Design review of the part built by this model. Coordinates are the model's own, in mm. Round coordinates to 2 decimals unless told otherwise and drop trailing zeros. Order: outer loops, then holes, each group sorted by start corner. A loop starts at its lowest first (then second) coordinate and runs counter-clockwise, first axis right, second up. Notation, with made-up numbers: (36, -1.5) - (41, -1.5) arc R21 ccw to (41, 2.5) - close; hole circle Ø3 at (-30, 40). An arc over 180 degrees is marked (long way). Write item = value, one per line.
from build123d import *

# Parameters (mm, degrees)
SKETCH_1_W                       = 385
SKETCH_1_H                       = 240
EXTRUDE_1_DEPTH                  = 16
SKETCH_2_R                       = 13.5
CUT_EXTRUDE_1_DEPTH              = 454.961452108
PATTERN_LINEAR_1_COUNT           = 2
PATTERN_LINEAR_1_PITCH           = 80
PATTERN_LINEAR_2_COUNT           = 2
PATTERN_LINEAR_2_PITCH           = 80
PATTERN_LINEAR_3_COUNT           = 2
PATTERN_LINEAR_3_PITCH           = 80
PATTERN_LINEAR_3_COPY_1_SKETCH_R = 13.5
PATTERN_LINEAR_3_COPY_1_DEPTH    = 454.961452108
PATTERN_LINEAR_3_COPY_2_SKETCH_R = 13.5
PATTERN_LINEAR_3_COPY_2_DEPTH    = 454.961452108
PATTERN_LINEAR_4_COUNT           = 2
PATTERN_LINEAR_4_PITCH           = 225
PATTERN_LINEAR_4_COPY_1_SKETCH_R = 13.5
PATTERN_LINEAR_4_COPY_1_DEPTH    = 454.961452108
PATTERN_LINEAR_4_COPY_2_SKETCH_R = 13.5
PATTERN_LINEAR_4_COPY_2_DEPTH    = 454.961452108
PATTERN_LINEAR_4_COPY_3_SKETCH_R = 13.5
PATTERN_LINEAR_4_COPY_3_DEPTH    = 454.961452108
PATTERN_LINEAR_4_COPY_4_SKETCH_R = 13.5
PATTERN_LINEAR_4_COPY_4_DEPTH    = 454.961452108
PATTERN_LINEAR_4_COPY_5_SKETCH_R = 13.5
PATTERN_LINEAR_4_COPY_5_DEPTH    = 454.961452108


with BuildPart() as part:
    # 草图1 → 凸台-拉伸1 (new body)
    with BuildSketch(Plane(origin=(0, 0, 0), x_dir=(1, 0, 0), z_dir=(0, 1, 0))):
        with Locations((192.5, 120)):
            Rectangle(SKETCH_1_W, SKETCH_1_H)
    extrude(amount=EXTRUDE_1_DEPTH)

    # 草图2 → 切除-拉伸1 (cut, through all)
    with BuildSketch(Plane(origin=(0, 16, 0), x_dir=(1, 0, 0), z_dir=(0, 1, 0))):
        with Locations(Location((120, 120, 0), (0, 0, 270))):
            Circle(SKETCH_2_R)
    cut_extrude_1 = extrude(amount=-CUT_EXTRUDE_1_DEPTH, mode=Mode.SUBTRACT)

    # 阵列(线性)1: 切除-拉伸1 ×2
    with Locations(*[(0, 0, -i * PATTERN_LINEAR_1_PITCH) for i in range(1, PATTERN_LINEAR_1_COUNT)]):
        add(cut_extrude_1, mode=Mode.SUBTRACT)

    # 阵列(线性)2: 切除-拉伸1 ×2
    with Locations(*[(0, 0, i * PATTERN_LINEAR_2_PITCH) for i in range(1, PATTERN_LINEAR_2_COUNT)]):
        add(cut_extrude_1, mode=Mode.SUBTRACT)

    # 阵列(线性)3: 切除-拉伸1 ×2
    with Locations(*[(-i * PATTERN_LINEAR_3_PITCH, 0, 0) for i in range(1, PATTERN_LINEAR_3_COUNT)]):
        add(cut_extrude_1, mode=Mode.SUBTRACT)

    # 阵列(线性)3 copy 1 sketch → 阵列(线性)3 copy 1 (cut, through all)
    with BuildSketch(Plane(origin=(-80, 16, -80), x_dir=(1, 0, 0), z_dir=(0, 1, 0))):
        with Locations(Location((120, 120, 0), (0, 0, 270))):
            Circle(PATTERN_LINEAR_3_COPY_1_SKETCH_R)
    extrude(amount=-PATTERN_LINEAR_3_COPY_1_DEPTH, mode=Mode.SUBTRACT)

    # 阵列(线性)3 copy 2 sketch → 阵列(线性)3 copy 2 (cut, through all)
    with BuildSketch(Plane(origin=(-80, 16, 80), x_dir=(1, 0, 0), z_dir=(0, 1, 0))):
        with Locations(Location((120, 120, 0), (0, 0, 270))):
            Circle(PATTERN_LINEAR_3_COPY_2_SKETCH_R)
    extrude(amount=-PATTERN_LINEAR_3_COPY_2_DEPTH, mode=Mode.SUBTRACT)

    # 阵列(线性)4: 切除-拉伸1 ×2
    with Locations(*[(i * PATTERN_LINEAR_4_PITCH, 0, 0) for i in range(1, PATTERN_LINEAR_4_COUNT)]):
        add(cut_extrude_1, mode=Mode.SUBTRACT)

    # 阵列(线性)4 copy 1 sketch → 阵列(线性)4 copy 1 (cut, through all)
    with BuildSketch(Plane(origin=(225, 16, -80), x_dir=(1, 0, 0), z_dir=(0, 1, 0))):
        with Locations(Location((120, 120, 0), (0, 0, 270))):
            Circle(PATTERN_LINEAR_4_COPY_1_SKETCH_R)
    extrude(amount=-PATTERN_LINEAR_4_COPY_1_DEPTH, mode=Mode.SUBTRACT)

    # 阵列(线性)4 copy 2 sketch → 阵列(线性)4 copy 2 (cut, through all)
    with BuildSketch(Plane(origin=(225, 16, 80), x_dir=(1, 0, 0), z_dir=(0, 1, 0))):
        with Locations(Location((120, 120, 0), (0, 0, 270))):
            Circle(PATTERN_LINEAR_4_COPY_2_SKETCH_R)
    extrude(amount=-PATTERN_LINEAR_4_COPY_2_DEPTH, mode=Mode.SUBTRACT)

    # 阵列(线性)4 copy 3 sketch → 阵列(线性)4 copy 3 (cut, through all)
    with BuildSketch(Plane(origin=(145, 16, 0), x_dir=(1, 0, 0), z_dir=(0, 1, 0))):
        with Locations(Location((120, 120, 0), (0, 0, 270))):
            Circle(PATTERN_LINEAR_4_COPY_3_SKETCH_R)
    extrude(amount=-PATTERN_LINEAR_4_COPY_3_DEPTH, mode=Mode.SUBTRACT)

    # 阵列(线性)4 copy 4 sketch → 阵列(线性)4 copy 4 (cut, through all)
    with BuildSketch(Plane(origin=(145, 16, -80), x_dir=(1, 0, 0), z_dir=(0, 1, 0))):
        with Locations(Location((120, 120, 0), (0, 0, 270))):
            Circle(PATTERN_LINEAR_4_COPY_4_SKETCH_R)
    extrude(amount=-PATTERN_LINEAR_4_COPY_4_DEPTH, mode=Mode.SUBTRACT)

    # 阵列(线性)4 copy 5 sketch → 阵列(线性)4 copy 5 (cut, through all)
    with BuildSketch(Plane(origin=(145, 16, 80), x_dir=(1, 0, 0), z_dir=(0, 1, 0))):
        with Locations(Location((120, 120, 0), (0, 0, 270))):
            Circle(PATTERN_LINEAR_4_COPY_5_SKETCH_R)
    extrude(amount=-PATTERN_LINEAR_4_COPY_5_DEPTH, mode=Mode.SUBTRACT)


solid = part.part
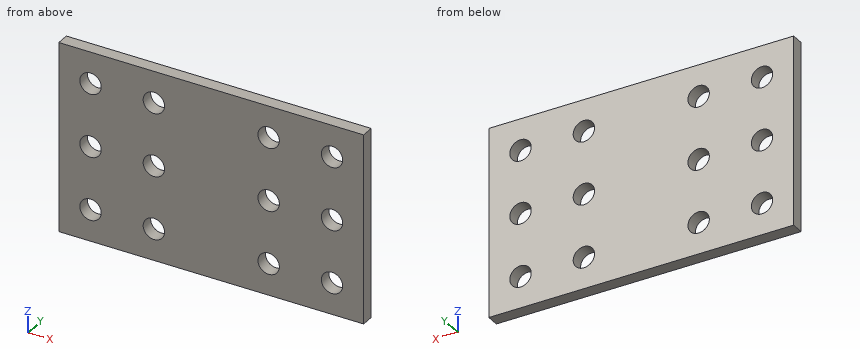
Item 1: Take a section at C-C, the plane x = 40. State the section outline as (y, z) points.
Data:
outline = (0, -240) - (16, -240) - (16, -213.5) - (0, -213.5) - close; (0, -186.5) - (16, -186.5) - (16, -133.5) - (0, -133.5) - close; (0, -106.5) - (16, -106.5) - (16, -53.5) - (0, -53.5) - close; (0, -26.5) - (16, -26.5) - (16, 0) - (0, 0) - close
Item 2: Take a section at A-A, the plane z = -120. State the section outline as (x, y) points, and give its area (3 significant figures).
Data:
outline = (0, 0) - (26.5, 0) - (26.5, 16) - (0, 16) - close; (53.5, 0) - (106.5, 0) - (106.5, 16) - (53.5, 16) - close; (133.5, 0) - (251.5, 0) - (251.5, 16) - (133.5, 16) - close; (278.5, 0) - (331.5, 0) - (331.5, 16) - (278.5, 16) - close; (358.5, 0) - (385, 0) - (385, 16) - (358.5, 16) - close
area = 4,430 mm2
Item 3: Take a section at B-B, the plane y = 4. Count the separate pieces of the cut face and the enclosed holes in it, and give its area (3 significant figures).
Data:
separate_pieces = 1
enclosed_holes = 12
area = 85,500 mm2
Item 4: Take a section at D-D, the plane x = 124.5. State the section outline as (y, z) points.
Data:
outline = (0, -240) - (16, -240) - (16, -212.73) - (0, -212.73) - close; (0, -187.27) - (16, -187.27) - (16, -132.73) - (0, -132.73) - close; (0, -107.27) - (16, -107.27) - (16, -52.73) - (0, -52.73) - close; (0, -27.27) - (16, -27.27) - (16, 0) - (0, 0) - close
Item 5: Insertion check: P1, Ø24.5, axis at x = 345, z = -40, coming from the -Y side; P2, Ø8, axis at x = 164.5, z = -116.5, coming from the -Y side. Each pin has a flat end and moves straight along its axis. Give the tip position at first contact, or say it passes through.
Data:
P1 = through
P2 = 0
Item 6: For line 1 along X through (y, z) = (9.5, -200); line 2 along Z through (x, y) = (252.5, 2.5), list the stretches that pass through material, from the lowest coordinate up. Write a range as [from, to].
Data:
line_1 = [0, 26.5], [53.5, 106.5], [133.5, 251.5], [278.5, 331.5], [358.5, 385]
line_2 = [-240, -205.1], [-194.9, -125.1], [-114.9, -45.1], [-34.9, 0]
